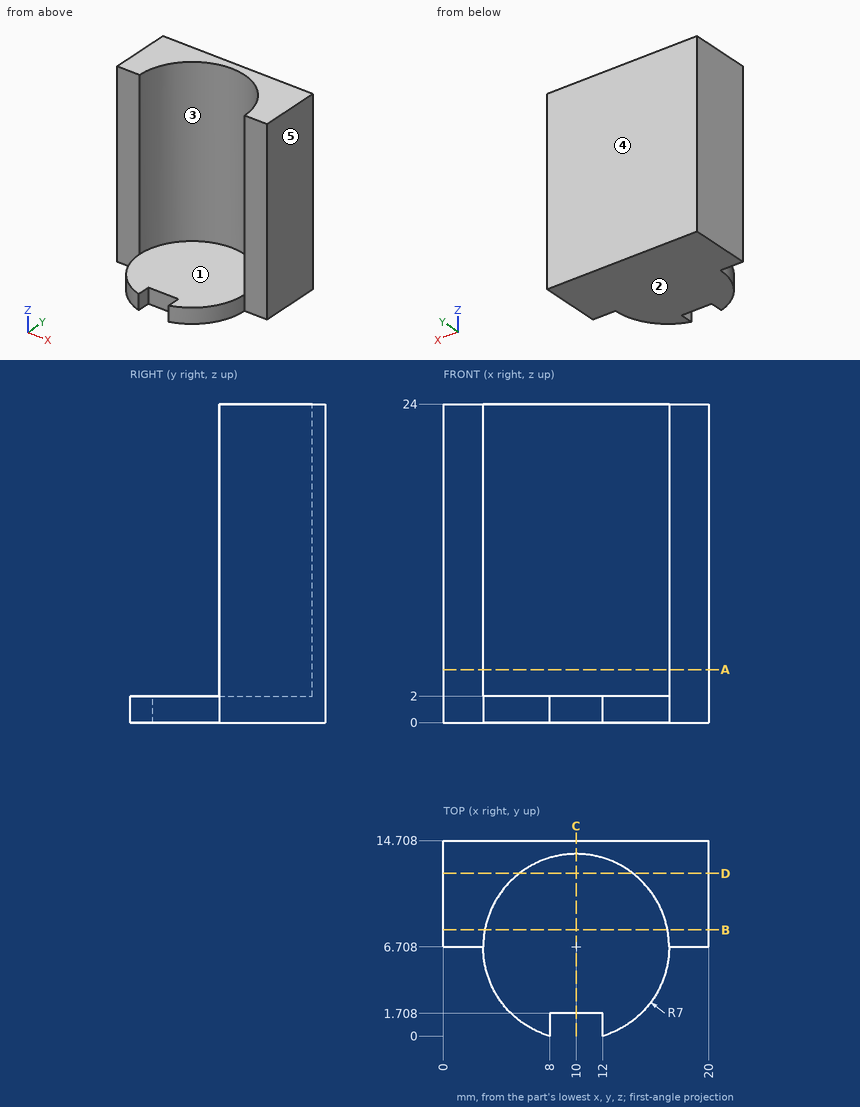
Here's the drawing with two shaded views (mm, measured from the low corner). I have some questions. A direction names the side the tool comes from. Give positions to 0.01 mm unless a question says otherwise; leave off trailing zeros. Loops run counter-clockwise (first coordinate to the right, second up) from the corner with the lowest first, then second, coordinate; pieces in that order, holes last. Notation, with made-up numbers: M 87.5,23.5 L 112.5,23.5 A18 cw 112.5,28.5 Z; hole C 74.5,11 d8. An arc over 180 degrees is marked long. One line per item, written item: value.
1) On a 3-axis mill with a long thin cutter (end or side, diameter ignored), from which of +Z, -Z, +X, -X, +Y, -Y can I reach the whole of each face in a straight line? I mean the marked faces 1 and 2. Say none if no direction works.
Geometry check:
face 1: +Z, -Y
face 2: -Z, +X, -X, +Y, -Y
2) I'm going to push flat-ended pins straight in: pin 1 (3.5 mm diameter, centred on x = 1.5, z = 7, fed in from -Y); pin 2 (0.5 mm diameter, centred on y = 1, z = 1.5, fed in from +X); pin 3 (4 mm diameter, centred on x = 8.5, y = 3.5, fed in from +Z). Where does each tip first touch, or does it pass through?
Geometry check:
pin 1: stops at y = 6.71
pin 2: stops at x = 14.38
pin 3: stops at z = 2
3) Imagine slicing it at C-C on x = 10. Write out the boundary of the cut face in (y, z).
Geometry check:
outline: M 1.71,0 L 14.71,0 L 14.71,24 L 13.71,24 L 13.71,2 L 1.71,2 Z
4) Imagine slicing it at D-D on y = 12.25. Write out the boundary of the cut face in (x, z).
Geometry check:
outline: M 0,0 L 20,0 L 20,24 L 14.28,24 L 14.28,2 L 5.72,2 L 5.72,24 L 0,24 Z
5) Imagine slicing it at A-A on z = 4. Write out the boundary of the cut face in (x, y).
Geometry check:
outline: M 0,6.71 L 3,6.71 A7 cw 17,6.71 L 20,6.71 L 20,14.71 L 0,14.71 Z
6) Please list where these lines run through material, in increasing order: line 1 (Z direction, x = 4.5, y = 2.75); line 2 (X direction, y = 8, z = 11.75); line 3 (X direction, y = 9.5, z = 3.5).
Geometry check:
line 1: z = 0 to 2
line 2: x = 0 to 3.12, 16.88 to 20
line 3: x = 0 to 3.58, 16.42 to 20
7) Thinking about a two-plate mould opening in X: for the marked faces 3, 4 and 5, which applies, +X half, -X half, draft (parallel to the pull), parting line (faces both ways), or undercut?
Geometry check:
face 3: undercut
face 4: draft
face 5: +X half
8) Imagine slicing it at B-B on y = 8. Write out the boundary of the cut face in (x, z).
Geometry check:
outline: M 0,0 L 20,0 L 20,24 L 16.88,24 L 16.88,2 L 3.12,2 L 3.12,24 L 0,24 Z
